Build history of the part. All positions in model axes, mm. Face numbers are marked on the shaded views. A direction names the side the tool comes from. Coordinates: 2 decimals unless noted, no trailing zeros. Write each loop counter-clockwise with the first axis right and the second up, starting at its lowest first coordinate (ties: lowest second). Pieces come first, ordered by that corner, then holes.
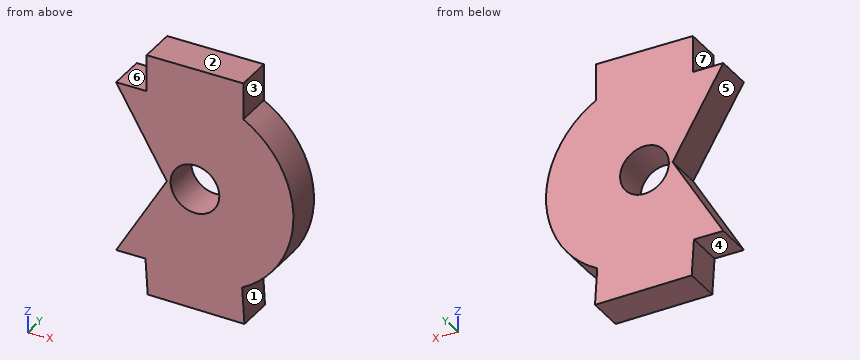
```python
from build123d import *

# Parameters (mm, degrees)
F0_R     = 3.2
F1_DEPTH = 4.826


with BuildPart() as f1:
    # F0 (on Front) → F1 (new body)
    with BuildSketch(Plane.XZ):
        with BuildLine():
            Line((-6.199785, -15.992633), (6.499093, -16.161406))
            Line((6.499093, -16.161406), (6.199785, -11.344696))
            ThreePointArc((6.199785, -11.344696), (12.927958, -0.085905), (6.35, 11.261304))
            Line((6.35, 11.261304), (6.35, 16.087304))
            Line((6.35, 16.087304), (-6.35, 16.087304))
            Line((-6.35, 16.087304), (-6.35, 11.261304))
            Line((-6.35, 11.261304), (-10.35, 11.261304))
            Line((-10.35, 11.261304), (-3.688663, -0.043395))
            Line((-3.688663, -0.043395), (-10.35, -11.261304))
            Line((-10.35, -11.261304), (-6.493788, -11.261304))
            Line((-6.493788, -11.261304), (-6.199785, -15.992633))
        make_face()
        Circle(F0_R, mode=Mode.SUBTRACT)
    extrude(amount=F1_DEPTH)


solid = f1.part
```
1. 3-axis set-ups, long thin cutter, end or side, ignore diameter. For the marked faces 1, 2 and 3: which of +Z, -Z, +X, -X, +Y, -Y reach the whole face in a straight line?
Computed values:
face 1: +X, +Y, -Y
face 2: +Z, +X, -X, +Y, -Y
face 3: +Z, +X, +Y, -Y
2. Saw through at D-D on z = -7.5. List the corners of the cut face in (x, y), plus the area to 3 significant figures.
Computed values:
outline: (-8.12, -4.83) - (10.53, -4.83) - (10.53, 0) - (-8.12, 0) - close
area: 90.0 mm2
3. Saw through at A-A on x = -5.25. List the corners of the cut face in (y, z), plus the area to 3 significant figures.
Computed values:
outline: (-4.83, -16.01) - (0, -16.01) - (0, -2.67) - (-4.83, -2.67) - close; (-4.83, 2.61) - (0, 2.61) - (0, 16.09) - (-4.83, 16.09) - close
area: 129 mm2
4. Mould opens along Z. For the marked faces 4, 5, 6 and 7 say: +Z half, -Z half, draft (parallel to the pull), parting line (faces both ways), or undercut.
Computed values:
face 4: -Z half
face 5: undercut
face 6: +Z half
face 7: draft
5. Saw through at B-B on y = -3.1. List the corners of the cut face in (x, z).
Computed values:
outline: (-10.35, -11.26) - (-6.49, -11.26) - (-6.2, -15.99) - (6.5, -16.16) - (6.2, -11.34) arc R12.93 ccw to (6.35, 11.26) - (6.35, 16.09) - (-6.35, 16.09) - (-6.35, 11.26) - (-10.35, 11.26) - (-3.69, -0.04) - close; hole circle Ø6.4 at (0, 0)
6. Flat gauge pins, fed straight in: pin 1 (2 mm diameter, centred on x = -1.5, z = -10, fed in from +Y); pin 2 (1.9 mm diameter, centred on x = -9.5, y = -3, fed in from -Z); pin 3 (2 mm diameter, centred on y = -2, z = -3, fed in from +X); pin 4 (6 mm diameter, centred on x = 0, z = 0, fed in from -Y). Where does each tip first touch, or does it go through?
Computed values:
pin 1: stops at y = 0
pin 2: stops at z = -11.26
pin 3: stops at x = 12.77
pin 4: passes through
7. Probe line 1 along X through (y, z) = (-3.05, 12); line 2 along Z through (x, y) = (0, -3.6); line 3 along Z through (x, y) = (-4.75, -3.3). List the from-to ranges inside material, lowest first.
Computed values:
line 1: x = -6.35 to 6.35
line 2: z = -16.08 to -3.2, 3.2 to 16.09
line 3: z = -16.01 to -1.83, 1.76 to 16.09
8. Saw through at C-C on x = 0. List the corners of the cut face in (y, z), plus the area to 3 significant figures.
Computed values:
outline: (-4.83, -16.08) - (0, -16.08) - (0, -3.2) - (-4.83, -3.2) - close; (-4.83, 3.2) - (0, 3.2) - (0, 16.09) - (-4.83, 16.09) - close
area: 124 mm2
